Could you check a few things on this model? Use its own coordinates, in mm. A direction names the side the tool comes from. Coordinates: 2 decimals unless noted, no trailing zeros. Write each loop counter-clockwise with the first axis right and the second up, starting at its lowest first coordinate (ties: lowest second). Pieces come first, ordered by that corner, then holes. Notation, with made-up numbers: (47, -9) - (77, -9) arc R25 ccw to (77, 15) - close; hole circle Ø2 at (59.5, 19). An arc over 180 degrees is marked (long way). Answer as a JSON object with one key per item and string values. Group by question number.
1) We'd pull the mould along Z, two halves only. Please class faces 1 (the flat face through (-0.49, -0.54, -0.87)), 2 (the flat face through (-1, 0, -1)), 3 (the cylindrical face through (-0.29, -1.19, 2.23)): released by +Z, released by -Z, zero draft, split by the parting line, or undercut.
2) Please list where these lines run through material, in increasing order: line 1 along Y through (x, z) = (-0.8, -0.4); line 2 along Y through (x, z) = (-1.1, -1.2); line 3 along Z through (x, y) = (0.1, -4.5).
3) If we section it at A-A (z = 0): Write out the boundary of the cut face in (x, y), plus the area to 3 significant figures.
4) Will these pins go through, and if not, where does the flat tip stop? pin 1 Ø0.6 at (x, z) = (0, 0) entering from +Y; pin 2 Ø1 at (y, z) = (-5, 0) entering from +X; pin 3 Ø2 at (x, y) = (-1.5, -4.5) entering from +Z.
5) If we section it at B-B (y = -1.5): Write out the boundary of the cut face in (x, z).
6) On a 3-axis mill with a long thin cutter (end or side, diameter ignored), from which of +Z, -Z, +X, -X, +Y, -Y can I reach the whole of each face in a straight line? I mean faces 4 (the flat face through (0, -1.1, 0)), 5 (the flat face through (0, -14.4, 0)), 6 (the flat face through (1, -2.4, 1)). Say none if no direction works.
```python
from build123d import *

# Parameters (mm, degrees)
SKETCH_1_W          = 2.25
SKETCH_1_H          = 2.4
SKETCH_2_R          = 1.25
EXTRUDE_1_DEPTH     = 12
CUT_EXTRUDE_1_DEPTH = 1.1
FILLET_1_R          = 0.3


with BuildPart() as part:
    # 草图1 → 旋转1 (revolve)
    with BuildSketch(Plane.XY):
        with Locations((1.125, -1.2)):
            Rectangle(SKETCH_1_W, SKETCH_1_H)
    revolve(axis=Axis((0, 0, 0), (0, -1, 0)))

    # 草图2 → 凸台-拉伸1 (add)
    with BuildSketch(Plane.XZ.offset(2.4)):
        with Locations(Location((0, 0, 0), (0, 0, 270))):
            Circle(SKETCH_2_R)
    extrude(amount=EXTRUDE_1_DEPTH)

    # 草图3 → 切除-拉伸1 (cut)
    with BuildSketch(Plane(origin=(0, 0, 0), x_dir=(-1, 0, 0), z_dir=(0, 1, 0))):
        Polygon((0, -1.154700538), (1, -0.577350269), (1, 0.577350269), (0, 1.154700538), (-1, 0.577350269), (-1, -0.577350269), align=None)
    extrude(amount=-CUT_EXTRUDE_1_DEPTH, mode=Mode.SUBTRACT)

    # 圆角1
    fillet_1_edges = [part.edges().sort_by_distance(p)[0] for p in [
        (0, -14.4, 1.25),
        (-2.25, -2.4, 0),
        (-2.25, 0, 0),
    ]]
    fillet(fillet_1_edges, radius=FILLET_1_R)


solid = part.part
```
Here are the results:
{
 "1": {"face 1": "undercut", "face 2": "zero draft", "face 3": "split by the parting line"},
 "2": {"line 1": "y = -14.4 to -1.1", "line 2": "y = -2.4 to 0", "line 3": "z = -1.25 to 1.25"},
 "3": {"outline": "(-2.25, -2.1) arc R0.3 ccw to (-1.95, -2.4) - (-1.25, -2.4) - (-1.25, -14.1) arc R0.3 ccw to (-0.95, -14.4) - (0.95, -14.4) arc R0.3 ccw to (1.25, -14.1) - (1.25, -2.4) - (1.95, -2.4) arc R0.3 ccw to (2.25, -2.1) - (2.25, -0.3) arc R0.3 ccw to (1.95, 0) - (1, 0) - (1, -1.1) - (-1, -1.1) - (-1, 0) - (-1.95, 0) arc R0.3 ccw to (-2.25, -0.3) - close", "area": "38.5 mm²"},
 "4": {"pin 1": "stops at y = -1.1", "pin 2": "stops at x = 1.25", "pin 3": "stops at z = 1.15"},
 "5": {"outline": "circle Ø4.5 at (0, 0)"},
 "6": {"face 4": "+Y", "face 5": "+Z, -Z, +X, -X, -Y", "face 6": "-Y"}
}
